Geometry check sheet. Reference: the model listing, model coordinates, mm. A direction names the side the tool comes from. Give positions to 0.01 mm unless a question says otherwise; leave off trailing zeros. Loops run counter-clockwise (first coordinate to the right, second up) from the corner with the lowest first, then second, coordinate; pieces in that order, holes last. Notation, with made-up numbers: (-21.5, 20) -> (33.5, 20) arc R22 ccw to (33.5, 40) -> close; hole circle Ø4 at (-27.75, 71). An arc over 180 degrees is marked (long way). Answer in a Markdown table with one row per item. Add a question column.
```python
from build123d import *

# Parameters (mm, degrees)
F1_DEPTH = 25.4
F2_W     = 27.981639
F2_H     = 12.533441
F3_DEPTH = 48.26
F4_R     = 7.874
F5_DEPTH = 52.324
F7_DEPTH = 48.514


with BuildPart() as f1:
    # F0 (on Front) → F1 (new body)
    with BuildSketch(Plane.XZ):
        Polygon((6.120985, 45.324426), (-43.104272, 8.321789), (-43.104272, -12.506211), (82.729638, -12.506211), (82.729638, 8.321789), (33.519674, 45.324426), align=None)
    extrude(amount=F1_DEPTH)

    # F2 (on Front) → F3 (join)
    with BuildSketch(Plane.XZ):
        with Locations((20.170395, 39.640653)):
            Rectangle(F2_W, F2_H)
    extrude(amount=F3_DEPTH)

    # F4 (on Top) → F5 (cut)
    with BuildSketch(Plane.XY):
        with Locations((19.295966, -37.45459)):
            Circle(F4_R)
    extrude(amount=F5_DEPTH, mode=Mode.SUBTRACT)

    # F6 (on Front) → F7 (join)
    with BuildSketch(Plane.XZ):
        Polygon((-8.696082, -5.683771), (-8.696082, -12.67918), (48.453918, -12.67918), (48.453918, -5.683771), (34.161214, 8.338805), (4.138858, 8.338805), align=None)
    extrude(amount=F7_DEPTH)


solid = f1.part
```
1. Sectioned sample at C-C (y = -18). Enter the section's corners in (x, z), plus the area to 3 significant figures.
2. Sectioned sample at A-A (y = -28). Enter the section's corners in (x, z).
3. Access from +Z, -Z, +X, -X, +Y, -Y to the whole of each face (thin tool, end or side, straight path). Record for faces 1 (the face through (6.18, -40, 40)), 2 (the face through (65, -13, -12.506)), 3 (the face through (20, -29, 33.374)), 4 (the face through (41.408, -36.795, 1.229)).
4. Material ranges on L1, parallel to Y at x = 10.5, z = 15.5; L2, parallel to Z at x = 10.5, y = -36; L3, parallel to Y at x = 20, z = 36.5, recorded low to high. Write a range as from..to.
5. Sectioned sample at D-D (z = 36). Enter the section's corners in (x, y).
6. Sectioned sample at B-B (x = 28.5). Enter the section's corners in (y, z), plus the area to 3 significant figures.
7. Gauge pin test, flat ends, axial feed: pin 1 Ø14 at (y, z) = (-35.5, 38) entering from +X; pin 2 Ø6 at (x, y) = (64.5, -6.5) entering from +Z; pin 3 Ø2 at (y, z) = (-30, -9.5) entering from +X. Record the tip position at first contact, or that the pin passes through.
8. Release check for a two-part mould opening along Y. For faces 5 (the face through (19, 0, 11)), 6 (the face through (48.454, -35, -9)), 7 (the face through (20, -48.26, 40)), 8 (the face through (22.93, -44.44, 39.55)) record: released by +Y, released by -Y, zero draft, split by the parting line, or undercut.
Response:
| question | item | result |
|---|---|---|
| 1 | outline | (-43.1, -12.51) -> (-8.7, -12.51) -> (-8.7, -12.68) -> (48.45, -12.68) -> (48.45, -12.51) -> (82.73, -12.51) -> (82.73, 8.32) -> (34.16, 44.84) -> (34.16, 45.91) -> (6.18, 45.91) -> (6.18, 45.32) -> (6.12, 45.32) -> (-43.1, 8.32) -> close |
| 1 | area | 5,480 mm2 |
| 2 | outline | (-8.7, -12.68) -> (48.45, -12.68) -> (48.45, -5.68) -> (34.16, 8.34) -> (4.14, 8.34) -> (-8.7, -5.68) -> close; (6.18, 33.37) -> (34.16, 33.37) -> (34.16, 45.91) -> (6.18, 45.91) -> close |
| 3 | face 1 | +Z, -X, -Y |
| 3 | face 2 | -Z, +X, +Y, -Y |
| 3 | face 3 | +X, -X, -Y |
| 3 | face 4 | +Z, +X, -Y |
| 4 | L1 | y = -25.4..0 |
| 4 | L2 | z = -12.68..8.34, 33.37..45.91 |
| 4 | L3 | y = -48.26..-45.3, -29.61..0 |
| 5 | outline | (-6.28, -25.4) -> (6.18, -25.4) -> (6.18, -48.26) -> (34.16, -48.26) -> (34.16, -25.4) -> (45.92, -25.4) -> (45.92, 0) -> (-6.28, 0) -> close; hole circle Ø15.75 at (19.3, -37.45) |
| 6 | outline | (-48.51, -12.68) -> (0, -12.68) -> (0, 45.91) -> (-48.26, 45.91) -> (-48.26, 33.37) -> (-25.4, 33.37) -> (-25.4, 8.34) -> (-48.51, 8.34) -> close |
| 6 | area | 2,260 mm2 |
| 7 | pin 1 | stops at x = 34.16 |
| 7 | pin 2 | stops at z = 24.29 |
| 7 | pin 3 | stops at x = 48.45 |
| 8 | face 5 | released by +Y |
| 8 | face 6 | zero draft |
| 8 | face 7 | released by -Y |
| 8 | face 8 | undercut |
